The listing builds one solid part. Answer for the finished solid, in the listing's coordinates (mm). A direction names the side the tool comes from. Round coordinates to 2 decimals unless told otherwise and drop trailing zeros. Loops run counter-clockwise (first coordinate to the right, second up) from the corner with the lowest first, then second, coordinate; pieces in that order, holes last. Notation, with made-up numbers: M 47.25,83 L 97.25,83 A16 ccw 97.25,100 Z; hole C 22,15.5 d4. An arc over 180 degrees is marked long. Answer as a JSON object with one key per item and string values.
```python
from build123d import *
from build123d.topology import SkipClean

# Parameters (mm, degrees)
ROTATION1_ANGLE                      = 180
SCHNITT_LINEAR_AUSTRAGEN2_DEPTH      = 92.33454987
SCHNITT_LINEAR_AUSTRAGEN2_DEPTH_BACK = 90
SCHNITT_LINEAR_AUSTRAGEN3_DEPTH      = 92.33454987
SCHNITT_LINEAR_AUSTRAGEN3_DEPTH_BACK = 90
SKIZZE8_W                            = 10
SKIZZE8_H                            = 5
AUFSATZ_LINEAR_AUSTRAGEN2_DEPTH      = 90
SKIZZE9_W                            = 10
SKIZZE9_H                            = 5
AUFSATZ_LINEAR_AUSTRAGEN3_DEPTH      = 90
SKIZZE12_R                           = 1
SCHNITT_LINEAR_AUSTRAGEN5_DEPTH      = 20
SKIZZE13_W                           = 38.761249726
SKIZZE13_H                           = 19.724182296
SCHNITT_LINEAR_AUSTRAGEN7_DEPTH      = 90
SKIZZE14_R                           = 4
SCHNITT_LINEAR_AUSTRAGEN8_DEPTH      = 5
SKIZZE15_R                           = 2
SCHNITT_LINEAR_AUSTRAGEN9_DEPTH      = 93.258379674
SKIZZE17_W                           = 21.457385309
SKIZZE17_H                           = 2
SCHNITT_LINEAR_AUSTRAGEN16_DEPTH     = 93.717898057


with BuildPart() as part:
    # Skizze3 → Rotation1 (revolve)
    with BuildSketch(Plane.XY):
        Polygon((0, 0), (-11, 0), (-11, 90), (-6, 90), (-6, 10), (0, 10), align=None)
    revolve(axis=Axis((0, 0, 0), (0, 1, 0)), revolution_arc=ROTATION1_ANGLE)

    # Skizze6 → Schnitt-Linear austragen2 (cut, two sides: drawn at the far end of the back side and taken through both)
    with BuildSketch(Plane(origin=(0, 90, 0), x_dir=(1, 0, 0), z_dir=(0, 1, 0)).offset(-SCHNITT_LINEAR_AUSTRAGEN2_DEPTH_BACK)):
        Polygon((-9.380624863, -62.0642209), (-9.380624863, -5.744900102), (-9.380624863, 0), (-9.380624863, 56.319320799), (-122.01926646, 56.319320799), (-122.01926646, -62.0642209), align=None)
    extrude(amount=SCHNITT_LINEAR_AUSTRAGEN2_DEPTH + SCHNITT_LINEAR_AUSTRAGEN2_DEPTH_BACK, mode=Mode.SUBTRACT)

    # Skizze7 → Schnitt-Linear austragen3 (cut, two sides: drawn at the far end of the back side and taken through both)
    with BuildSketch(Plane.XZ.offset(-SCHNITT_LINEAR_AUSTRAGEN3_DEPTH_BACK)):
        Polygon((9.380624863, 59.241313346), (9.380624863, 5.744900102), (9.380624863, 0), (9.380624863, -53.496413245), (116.373451353, -53.496413245), (116.373451353, 59.241313346), align=None)
    extrude(amount=SCHNITT_LINEAR_AUSTRAGEN3_DEPTH + SCHNITT_LINEAR_AUSTRAGEN3_DEPTH_BACK, mode=Mode.SUBTRACT)

    # Skizze8 → Aufsatz-Linear austragen2 (add)
    with BuildSketch(Plane(origin=(0, 90, 0), x_dir=(1, 0, 0), z_dir=(0, 1, 0))):
        with Locations((-14.380624863, -2.5)):
            Rectangle(SKIZZE8_W, SKIZZE8_H)
    extrude(amount=-AUFSATZ_LINEAR_AUSTRAGEN2_DEPTH)

    # Skizze9 → Aufsatz-Linear austragen3 (add)
    with BuildSketch(Plane(origin=(0, 90, 0), x_dir=(1, 0, 0), z_dir=(0, 1, 0))):
        with Locations((14.380624863, -2.5)):
            Rectangle(SKIZZE9_W, SKIZZE9_H)
    extrude(amount=-AUFSATZ_LINEAR_AUSTRAGEN3_DEPTH)

    # Skizze12 → Schnitt-Linear austragen5 (cut)
    with BuildSketch(Plane(origin=(0, 0, 0), x_dir=(-1, 0, 0), z_dir=(0, -1, 0))):
        Circle(SKIZZE12_R)
    extrude(amount=-SCHNITT_LINEAR_AUSTRAGEN5_DEPTH, mode=Mode.SUBTRACT)

    # Spiegeln2: part across face


with BuildPart() as part_1:
    with SkipClean():  # the faces are left unmerged after this step: merging them gives an invalid solid
        add(part.part)
        add(part.part.mirror(Plane(origin=(12.323947404, 43.405429497, 0), x_dir=(1, 0, 0), z_dir=(0, 0, -1))))

    # Skizze13 → Schnitt-Linear austragen7 (cut)
    with BuildSketch(Plane(origin=(0, 0, 0), x_dir=(-1, 0, 0), z_dir=(0, -1, 0))):
        with Locations((0, -9.862091148)):
            Rectangle(SKIZZE13_W, SKIZZE13_H)
    extrude(amount=-SCHNITT_LINEAR_AUSTRAGEN7_DEPTH, mode=Mode.SUBTRACT)

    # Skizze14 → Schnitt-Linear austragen8 (cut)
    with BuildSketch(Plane(origin=(0, 0, 0), x_dir=(-1, 0, 0), z_dir=(0, -1, 0))):
        Circle(SKIZZE14_R)
    extrude(amount=-SCHNITT_LINEAR_AUSTRAGEN8_DEPTH, mode=Mode.SUBTRACT)

    # Skizze15 → Schnitt-Linear austragen9 (cut, through all)
    with BuildSketch(Plane(origin=(0, 0, -5), x_dir=(-1, 0, 0), z_dir=(0, 0, -1))):
        with Locations((-14.380624863, 80)):
            Circle(SKIZZE15_R)
        with Locations((-14.392959085, 10)):
            Circle(SKIZZE15_R)
        with Locations((14.380624863, 10)):
            Circle(SKIZZE15_R)
        with Locations((14.380624863, 80)):
            Circle(SKIZZE15_R)
    extrude(amount=-SCHNITT_LINEAR_AUSTRAGEN9_DEPTH, mode=Mode.SUBTRACT)

    # Skizze17 → Schnitt-Linear austragen16 (cut, through all)
    with BuildSketch(Plane(origin=(0, 90, 0), x_dir=(1, 0, 0), z_dir=(0, 1, 0))):
        with Locations((0.273845189, 10.009257492)):
            Rectangle(SKIZZE17_W, SKIZZE17_H)
    extrude(amount=-SCHNITT_LINEAR_AUSTRAGEN16_DEPTH, mode=Mode.SUBTRACT)


solid = part_1.part
```
Item 1: Determine the mould class of faces 6 (the face through (0, 49, -6)), 7 (the face through (-14.12, 81.983, -2.535)), 8 (the face through (15.87, 11.35, -2.54)), 9 (the face through (-0.3, 0, -4.4)) for opening direction Y: released by +Y, released by -Y, zero draft, split by the parting line, or undercut.
Values follow:
{"face 6": "zero draft", "face 7": "undercut", "face 8": "undercut", "face 9": "released by -Y"}
Item 2: The part is cut by section A-A (y = 80). Give the vertices of the cut face in (x, z), then the cut area to 3 significant figures.
Values follow:
{"outline": "M -19.38,-5 L -16.38,-5 L -16.38,0 L -19.38,0 Z; M -12.38,-5 L -9.38,-5 L -9.38,-5.74 A11 ccw -6.31,-9.01 L 6.31,-9.01 A11 ccw 9.38,-5.74 L 9.38,-5 L 12.38,-5 L 12.38,0 L 6,0 A6 cw -6,0 L -12.38,0 Z; M 16.38,-5 L 19.38,-5 L 19.38,0 L 16.38,0 Z", "area": "164 mm^2"}
Item 3: The part is cut by section D-D (x = 0). Give the vertices of the cut face in (y, z), then the cut area to 3 significant figures.
Values follow:
{"outline": "M 0,-9.01 L 90,-9.01 L 90,-6 L 10,-6 L 10,-1 L 5,-1 L 5,-4 L 0,-4 Z", "area": "306 mm^2"}
Item 4: Flat-ended cylindrical pins translate along their axes: P1, Ø4.5, axis at x = 14.39, y = 10, coming from the -Z side; P2, Ø3, axis at x = 2.5, z = -3.5, coming from the +Y side; P3, Ø1.2, axis at x = 0.5, z = -1.5, coming from the -Y side. Find the tip coordinate at first contact, or state that the pin passes through.
Values follow:
{"P1": "z = -5", "P2": "y = 10", "P3": "y = 5"}
Item 5: The part is cut by section C-C (y = 18). Give the vertices of the cut face in (x, z), then the cut area to 3 significant figures.
Values follow:
{"outline": "M -19.38,-5 L -9.38,-5 L -9.38,-5.74 A11 ccw -6.31,-9.01 L 6.31,-9.01 A11 ccw 9.38,-5.74 L 9.38,-5 L 19.38,-5 L 19.38,0 L 6,0 A6 cw -6,0 L -19.38,0 Z", "area": "204 mm^2"}
Item 6: Straight lines are drawn through the part: line 1 (Y direction, x = 13, z = -0.25); line 2 (Z direction, x = 17, y = 24.5); line 3 (X direction, y = 18, z = -4.5). For each, find the intervals that lie inside material, in ascending order.
Values follow:
{"line 1": "0 to 8.56, 11.44 to 78.55, 81.45 to 90", "line 2": "-5 to 0", "line 3": "-19.38 to -3.97, 3.97 to 19.38"}
Item 7: The part is cut by section B-B (x = 15). Give the vertices of the cut face in (y, z), then the cut area to 3 significant figures.
Values follow:
{"outline": "M 0,-5 L 8.09,-5 L 8.09,0 L 0,0 Z; M 11.91,-5 L 78.1,-5 L 78.1,0 L 11.91,0 Z; M 81.9,-5 L 90,-5 L 90,0 L 81.9,0 Z", "area": "412 mm^2"}
Item 8: Which of the six approach directions +Z, -Z, +X, -X, +Y, -Y give full straight-line access (tool end or side, diameter ignored) to faces 1 (the face through (0, 5, -2)), 2 (the face through (14, 46, -5)), 3 (the face through (-15.456, 11.686, -2.535)), 4 (the face through (0, 10, -2)), 5 (the face through (-12, 44, 0))?
Values follow:
{"face 1": "+Z, -Y", "face 2": "-Z, +X, +Y, -Y", "face 3": "+Z, -Z", "face 4": "+Z, +Y", "face 5": "+Z, +X, -X, +Y, -Y"}
